Input: dimensioned drawing with shaded views. Units: mm. Origin: part minimum x, y, z. A direction names the side the tool comes from. Coordinates: 2 decimals unless noted, no trailing zeros. Loops run counter-clockwise (first coordinate to the right, second up) from the corner with the lowest first, then second, coordinate; pieces in that order, holes last. Notation, with made-up numbers: M 64,14.25 L 74,14.25 A29 cw 74,43.25 Z; hole C 84.25,85 d3. An arc over 180 degrees is marked long. Write item = value, one per line. Start each with the question number.
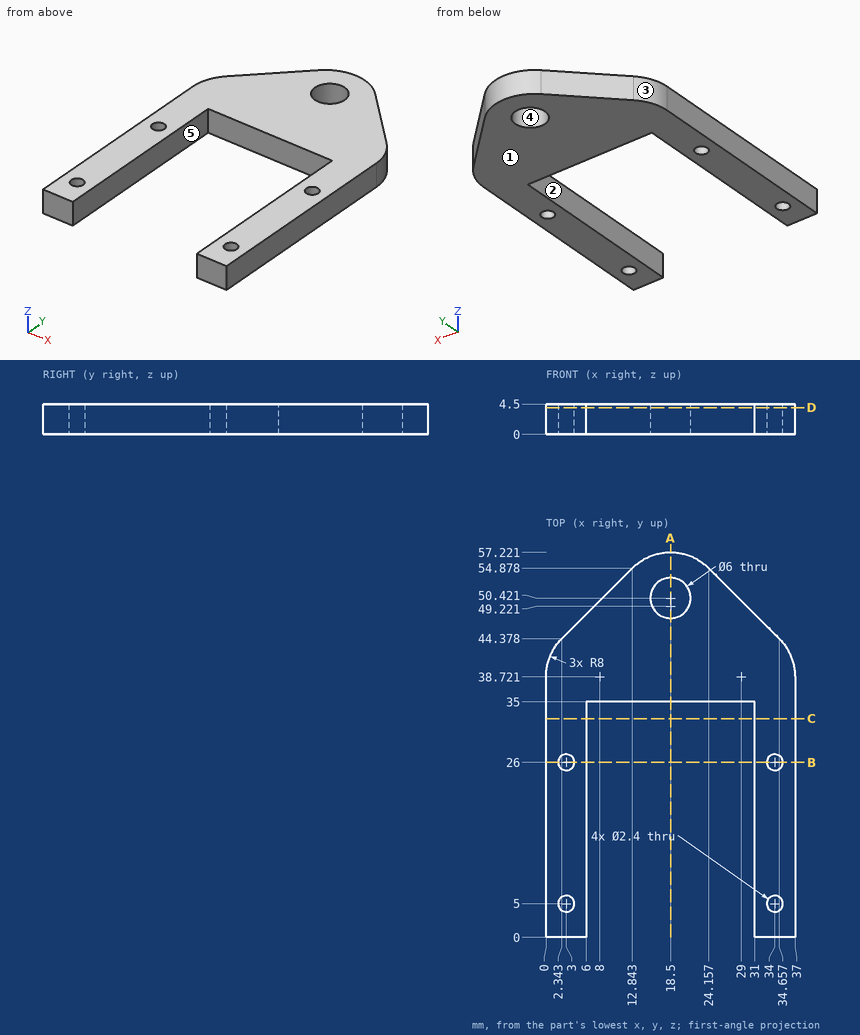
Item 1: Section query B-B (y = 26). Return the cut outline in (x, z).
Item 2: Reachability of the marked faces 1 and 2 from +Z, -Z, +X, -X, +Y, -Y: full face, straight path, thin tool, end or side. Return the list, or none.
Item 3: Section query D-D (z = 3.95). Return the cut outline in (x, y).
Item 4: First-contact query: pin 1 (1.9 mm diameter, centred on x = 3, y = 26, fed in from -Z); pin 2 (2 mm diameter, centred on y = 18, z = 3, fed in from -X); pin 3 (1 mm diameter, centred on x = 32.5, z = 1, fed in from +Y) (1 decimal). Flat tips, straight axial feed; report the tip coordinate or a pass-through.
Item 5: Pull-direction query (Y, two-part tool) for the marked faces 3, 4 and 5; classes: released by +Y, released by -Y, zero draft, split by the parting line, or undercut.
Item 6: Section query C-C (y = 32.5). Return the cut outline in (x, z).
Item 7: Line query: line 1 (X direction, y = 16.5, z = 4.3); line 2 (Y direction, x = 34, z = 2.05) (1 decimal); line 3 (X direction, y = 52.5, z = 0.8) (1 decimal). Output: solid intervals per line, ascending. Write a range as from..to.
Item 8: Section query A-A (x = 18.5). Return the cut outline in (y, z), plus the area to 3 significant figures.
Verdict:
q1.outline = M 0,0 L 1.8,0 L 1.8,4.5 L 0,4.5 Z; M 4.2,0 L 6,0 L 6,4.5 L 4.2,4.5 Z; M 31,0 L 32.8,0 L 32.8,4.5 L 31,4.5 Z; M 35.2,0 L 37,0 L 37,4.5 L 35.2,4.5 Z
q2.face_1 = -Z, +X, -X, +Y, -Y
q2.face_2 = +Z, -Z, -Y
q3.outline = M 0,0 L 6,0 L 6,35 L 31,35 L 31,0 L 37,0 L 37,38.72 A8 ccw 34.66,44.38 L 24.16,54.88 A8 ccw 12.84,54.88 L 2.34,44.38 A8 ccw 0,38.72 Z; hole C 3,5 d2.4; hole C 3,26 d2.4; hole C 18.5,50.42 d6; hole C 34,5 d2.4; hole C 34,26 d2.4
q4.pin_1 = through
q4.pin_2 = 0
q4.pin_3 = 47
q5.face_3 = released by +Y
q5.face_4 = undercut
q5.face_5 = zero draft
q6.outline = M 0,0 L 6,0 L 6,4.5 L 0,4.5 Z; M 31,0 L 37,0 L 37,4.5 L 31,4.5 Z
q7.line_1 = 0..6, 31..37
q7.line_2 = 0..3.8, 6.2..24.8, 27.2..45
q7.line_3 = 10.5..16.3, 20.7..26.5
q8.outline = M 35,0 L 47.42,0 L 47.42,4.5 L 35,4.5 Z; M 53.42,0 L 57.22,0 L 57.22,4.5 L 53.42,4.5 Z
q8.area = 73.0 mm2
